Could you check a few things on this model? Use its own coordinates, in mm. A direction names the side the tool comes from. Round coordinates to 2 decimals unless told otherwise and drop trailing zeros. Order: outer loops, then holes, each group sorted by start corner. A loop starts at its lowest first (then second) coordinate and runs counter-clockwise, first axis right, second up. Notation, with made-up numbers: (-3, 80) - (49, 80) arc R17 cw to (49, 93) - close; hole circle Ø5 at (10, 23). An arc over 180 degrees is marked (long way). Return JSON: item names as keys, results as strings. Group by question number.
from build123d import *

# Parameters (mm, degrees)
RESSALTO_EXTRUS_O1_DEPTH   = 2
RESSALTO_EXTRUS_O1_2_DEPTH = 2
ESBO_O2_R                  = 50
ESBO_O2_R_2                = 45
RESSALTO_EXTRUS_O2_DEPTH   = 10


with BuildPart() as part:
    # Esbo_o1 → Ressalto-extrus_o1 (new body)
    with BuildSketch(Plane.XY):
        with BuildLine():
            Line((-64.194703831, 10.2), (-10.998181668, 10.2))
            ThreePointArc((-10.998181668, 10.2), (0, 15), (10.998181668, 10.2))
            Line((10.998181668, 10.2), (64.194703831, 10.2))
            ThreePointArc((64.194703831, 10.2), (0, 65), (-64.194703831, 10.2))
        make_face()
    extrude(amount=RESSALTO_EXTRUS_O1_DEPTH)



with BuildPart() as body_2:
    # Esbo_o1 → Ressalto-extrus_o1 2 (new body)
    with BuildSketch(Plane.XY):
        with BuildLine():
            Line((-10.998181668, -10.2), (-64.194703831, -10.2))
            ThreePointArc((-64.194703831, -10.2), (0, -65), (64.194703831, -10.2))
            Line((64.194703831, -10.2), (10.998181668, -10.2))
            ThreePointArc((10.998181668, -10.2), (0, -15), (-10.998181668, -10.2))
        make_face()
    extrude(amount=RESSALTO_EXTRUS_O1_2_DEPTH)


with BuildPart() as part_1:
    add(part.part)

    add(body_2.part)  # Ressalto-extrus_o2 merges body 2
    # Esbo_o2 → Ressalto-extrus_o2 (add)
    with BuildSketch(Plane.XY):
        with Locations(Location((0, 0, 0), (0, 0, 168.229033732))):
            Circle(ESBO_O2_R)
        with Locations(Location((0, 0, 0), (0, 0, 166.899096466))):
            Circle(ESBO_O2_R_2, mode=Mode.SUBTRACT)
    extrude(amount=RESSALTO_EXTRUS_O2_DEPTH)


solid = part_1.part
1) Will these pins go through, and if not, where does the flat tip stop? pin 1 (0.6 mm diameter, centred on x = -21, z = 1, fed in from +Y); pin 2 (5 mm diameter, centred on y = 34, z = 2.5, fed in from -X); pin 3 (1 mm diameter, centred on x = 31, z = 1, fed in from +Y); pin 4 (1 mm diameter, centred on x = -51, z = 8, fed in from +Y).
2) I want a section at B-B, the plane x = 0. List the corners of the cut face in (y, z) for me, plus the area to 3 significant figures.
3) I want a section at A-A, the plane y = 0. List the corners of the cut face in (x, z) for me, plus the area to 3 significant figures.
4) For faces 1 (the flat face through (4, -52, 2)), 2 (the flat face through (-1, 24, 2)), 3 (the cylindrical face through (0, 15, 1)), which set-ups out of +Z, -Z, +X, -X, +Y, -Y let a thin tool reach every point of the face, with its end or its side?
5) If I drill on line 1 along X through (y, z) = (0, 4.75); line 2 along Z through (x, y) = (-49, 27), over which ranges is the centre line in solid material (lowest first)? Write a range as from..to.
6) I want a section at D-D, the plane y = -16.5. List the corners of the cut face in (x, z) for me.
7) I want a section at C-C, the plane z = 5.5. List the corners of the cut face in (x, y) for me, plus the area to 3 significant figures.
Outcome:
{
 "1": {"pin 1": "y = 61.62", "pin 2": "x = -56.83", "pin 3": "y = 57.4", "pin 4": "through"},
 "2": {"outline": "(-65, 0) - (-15, 0) - (-15, 2) - (-45, 2) - (-45, 10) - (-50, 10) - (-50, 2) - (-65, 2) - close; (15, 0) - (65, 0) - (65, 2) - (50, 2) - (50, 10) - (45, 10) - (45, 2) - (15, 2) - close", "area": "280 mm^2"},
 "3": {"outline": "(-50, 0) - (-45, 0) - (-45, 10) - (-50, 10) - close; (45, 0) - (50, 0) - (50, 10) - (45, 10) - close", "area": "100 mm^2"},
 "4": {"face 1": "+Z, -Y", "face 2": "+Z", "face 3": "+Z, -Z"},
 "5": {"line 1": "-50..-45, 45..50", "line 2": "0..2"},
 "6": {"outline": "(-62.87, 0) - (62.87, 0) - (62.87, 2) - (47.2, 2) - (47.2, 10) - (41.87, 10) - (41.87, 2) - (-41.87, 2) - (-41.87, 10) - (-47.2, 10) - (-47.2, 2) - (-62.87, 2) - close"},
 "7": {"outline": "circle Ø100 at (0, 0); hole circle Ø90 at (0, 0)", "area": "1,490 mm^2"}
}
